Verification items for the finished model (mm, model axes). Round coordinates to 2 decimals unless told otherwise and drop trailing zeros. Write each loop counter-clockwise with the first axis right and the second up, starting at its lowest first coordinate (ties: lowest second). Pieces come first, ordered by that corner, then holes. Notation, with made-up numbers: (-36.75, -27.5) - (-13.75, -27.5) arc R17 ccw to (-13.75, 4.5) - close; hole circle Ø5 at (72, -13). An arc over 180 degrees is marked (long way). Write each question's results on one line, items separated by ' | '.
Autodesk Fusion 360 part; units mm, degrees
sketch "Sketch1" plane through (0, 0, 0) normal (0, 0, 1) x (1, 0, 0)
  line L0 (27, 38) -> (-27, 38)
  line L1 (-27, 38) -> (-27, -38)
  line L2 (-27, -38) -> (27, -38)
  line L3 (27, -38) -> (27, 38)
  line L4 (27, 38) -> (-27, -38) construction
  line L5 (-27, 38) -> (27, -38) construction
  line L6 (-27, 30) -> (27, 30)
  line L7 (0, 0) -> (5, 0)
  line L8 (0, 0) -> (0, 6)
  line L9 (-27, -30) -> (27, -30)
  line L10 (-12.5, 30) -> (-12.5, -30)
  line L11 (12.5, 30) -> (12.5, -30)
  line L12 (-12.5, 30) -> (-12.5, 38)
  line L13 (12.5, 30) -> (12.5, 38)
  circle A0 centre (0, 33) radius 1.7
  circle A1 centre (0, -33) radius 1.7
  line L14 (-12.5, -30) -> (-12.5, -38)
  line L15 (12.5, -30) -> (12.5, -38)
  circle A2 centre (-20.55, 33) radius 1.7
  circle A3 centre (-6.55, 33) radius 1.7
  circle A4 centre (20.55, 33) radius 1.7
  circle A5 centre (6.55, 33) radius 1.7
  circle A6 centre (-20.55, -33) radius 1.7
  circle A7 centre (-6.55, -33) radius 1.7
  circle A8 centre (6.55, -33) radius 1.7
  circle A9 centre (20.55, -33) radius 1.7
  dimension "d1" = 8
  dimension "d2" = 25
  dimension "d3" = 25
  dimension "d5" = 5
  dimension "d6" = 3.4
  dimension "d9" = 14
  dimension "d10" = 20.55
  dimension "d13" = 60
  dimension "d14" = 54
extrude "Extrude1" add sketch "Sketch1" along normal blind 2 contours L0 L6 L12 L13 | L6 L9 L10 L11 | L2 L9 L14 L15
equation "d10 = ( 41.1 / 2 ) * 1 mm"
(1) Go/stop test with a flat-tipped pin: pin 1 Ø2 at (x, y) = (6.55, -33) entering from +Z. Record where the tip stops, or that it passes through.
Answer:
pin 1: through
(2) Section check C-C (z = 1.55). Record the cut outline in (x, y), plus the area to 3 significant figures.
Answer:
outline: (-12.5, -38) - (12.5, -38) - (12.5, 38) - (-12.5, 38) - close; hole circle Ø3.4 at (-6.55, -33); hole circle Ø3.4 at (-6.55, 33); hole circle Ø3.4 at (0, -33); hole circle Ø3.4 at (0, 33); hole circle Ø3.4 at (6.55, -33); hole circle Ø3.4 at (6.55, 33) | area: 1,850 mm2
(3) Section check B-B (y = 33). Record the cut outline in (x, z), plus the area to 3 significant figures.
Answer:
outline: (-12.5, 0) - (-8.25, 0) - (-8.25, 2) - (-12.5, 2) - close; (-4.85, 0) - (-1.7, 0) - (-1.7, 2) - (-4.85, 2) - close; (1.7, 0) - (4.85, 0) - (4.85, 2) - (1.7, 2) - close; (8.25, 0) - (12.5, 0) - (12.5, 2) - (8.25, 2) - close | area: 29.6 mm2
(4) Section check D-D (x = -0.5). Record the cut outline in (y, z).
Answer:
outline: (-38, 0) - (-34.62, 0) - (-34.62, 2) - (-38, 2) - close; (-31.38, 0) - (31.38, 0) - (31.38, 2) - (-31.38, 2) - close; (34.62, 0) - (38, 0) - (38, 2) - (34.62, 2) - close
(5) Section check A-A (x = 5.75). Record the cut outline in (y, z), plus the area to 3 significant figures.
Answer:
outline: (-38, 0) - (-34.5, 0) - (-34.5, 2) - (-38, 2) - close; (-31.5, 0) - (31.5, 0) - (31.5, 2) - (-31.5, 2) - close; (34.5, 0) - (38, 0) - (38, 2) - (34.5, 2) - close | area: 140 mm2
(6) Thickness scan on L1, parallel to Y at x = 0, z = 0.5; L2, parallel to X at y = 34.5, z = 1; L3, parallel to Y at x = -7.25, z = 0.55. Record the ranges inside material, lowest first.
Answer:
L1: -38 to -34.7, -31.3 to 31.3, 34.7 to 38 | L2: -12.5 to -7.35, -5.75 to -0.8, 0.8 to 5.75, 7.35 to 12.5 | L3: -38 to -34.55, -31.45 to 31.45, 34.55 to 38
(7) Mould release check, pull along X, two halves, no side actions. Record for faces 1 (the cylindrical face through (6.18, 34.66, 0.99)), 2 (the flat face through (-12.5, -1, 1)), 3 (the flat face through (0, 38, 1)): released by +X, released by -X, zero draft, split by the parting line, or undercut.
Answer:
face 1: undercut | face 2: released by -X | face 3: zero draft
